Could you check a few things on this model? Use its own coordinates, in mm. Face numbers are marked on the shaded views. A direction names the side the tool comes from. Coordinates: 2 decimals unless noted, no trailing zeros. Loops run counter-clockwise (first coordinate to the right, second up) from the corner with the lowest first, then second, coordinate; pieces in that order, holes last. Notation, with made-up numbers: (26, 11.25) -> (43, 11.25) arc R7 cw to (43, 19.25) -> close; hole circle Ø4 at (25, 15). An arc over 180 degrees is marked (long way). One line per question, with ' | ' between items. Start each with the question number.
(1) Suppose I cut it at A-A (x = 17.5). Please give me the cut outline in (y, z).
(2) Suppose I cut it at C-C (y = -14). Please give me the cut outline in (x, z), plus the area to 3 significant figures.
(3) I'm going to push flat-ended pins straight in: pin 1 Ø1 at (x, y) = (62, -45.5) entering from +Z; pin 2 Ø19 at (x, y) = (15.5, -23) entering from +Z; pin 3 Ø5 at (y, z) = (-31, 35.5) entering from +X. Where does each tip first touch, or does it pass through?
(4) If I drill on line 1 along Z through (x, y) = (21, -42.5); line 2 along X through (y, z) = (-48, 21); line 3 along Y through (x, z) = (55, 30), over which ranges is the centre line in solid material (lowest first)?
(5) Suppose I cut it at D-D (x = 61). Please give me the cut outline in (y, z), plus the area to 3 significant figures.
(6) Suppose I cut it at B-B (z = 27). Please give me the cut outline in (x, y).
(7) If we mould it in two halves opening along Y, with no side actions, what happens to the marked faces 1, 2 and 3? For each: pulls with the +Y half, pulls with the -Y half, needs draft (parallel to the pull), parting line crosses it, or undercut.
(8) Which directions (+Z, -Z, +X, -X, +Y, -Y) give clear straight access to the entire face, cutting with the end or side of a thin tool? Please do the marked faces 4, 5 and 6.
```python
from build123d import *

# Parameters (mm, degrees)
F1_DEPTH = 50.8
F2_DEPTH = 12.7
F3_R     = 3.771706
F4_DEPTH = 127


with BuildPart() as f1:
    # F0 (on Front) → F1 (new body)
    with BuildSketch(Plane.XZ):
        Polygon((43.533504, 41.975465), (0, 41.975465), (0, 0), (66.480095, 0), align=None)
    extrude(amount=F1_DEPTH)

    # F0 (on Front) → F2 (join)
    with BuildSketch(Plane.XZ):
        Polygon((43.533504, 54.989692), (0, 54.989692), (0, 41.975465), (43.533504, 41.975465), (66.480095, 0), (73.59454, 0), align=None)
    extrude(amount=F2_DEPTH)

    # F3 (on face) → F4 (cut, symmetric)
    with BuildSketch(Plane(origin=(0, 0, 0), x_dir=(0, -1, 0), z_dir=(-1, 0, 0))):
        with Locations((32.626301, 22.3139)):
            Circle(F3_R)
    extrude(amount=F4_DEPTH, both=True, mode=Mode.SUBTRACT)


solid = f1.part
```
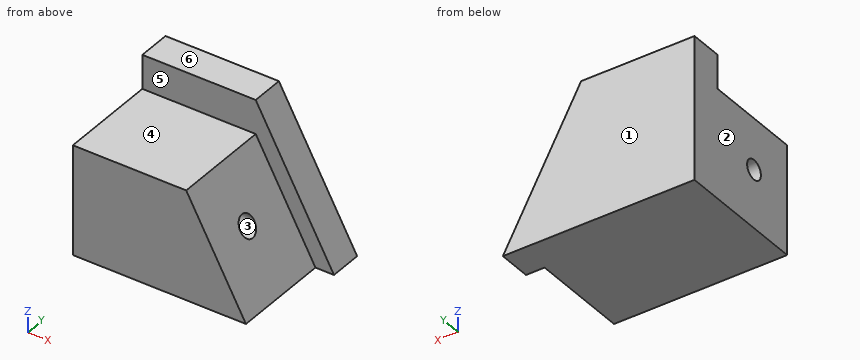
Checks:
1) outline: (-50.8, 0) -> (0, 0) -> (0, 54.99) -> (-12.7, 54.99) -> (-12.7, 41.98) -> (-50.8, 41.98) -> close; hole circle Ø7.54 at (-32.63, 22.31)
2) outline: (0, 0) -> (66.48, 0) -> (43.53, 41.98) -> (0, 41.98) -> close | area: 2,310 mm^2
3) pin 1: stops at z = 9.11 | pin 2: stops at z = 41.98 | pin 3: stops at x = 48.44
4) line 1: z = 0 to 41.98 | line 2: x = 0 to 55 | line 3: y = -12.7 to 0
5) outline: (-50.8, 0) -> (0, 0) -> (0, 23.04) -> (-12.7, 23.04) -> (-12.7, 10.02) -> (-50.8, 10.02) -> close | area: 675 mm^2
6) outline: (0, -50.8) -> (51.72, -50.8) -> (51.72, -12.7) -> (58.83, -12.7) -> (58.83, 0) -> (0, 0) -> close
7) face 1: pulls with the +Y half | face 2: needs draft | face 3: undercut
8) face 4: +Z, +X, -X, -Y | face 5: +Z, +X, -Y | face 6: +Z, +X, -X, +Y, -Y
